```python
from build123d import *

# Parameters (mm, degrees)
F1_DEPTH = 22
F2_R     = 6
F3_W     = 66
F3_H     = 4
F4_DEPTH = 96
F5_R     = 4.6734146419
F5_R_2   = 4.6518685429
F5_R_3   = 4.696387476
F5_R_4   = 4.5347148874
F5_R_5   = 2.5803932982
F5_R_6   = 2.1193315606
F5_R_7   = 2.8799856964
F5_R_8   = 3.6433218135
F5_R_9   = 1.5618927534
F5_R_10  = 1.780828752
F5_R_11  = 1.3177092187
F5_R_12  = 1.8635222484
F5_R_13  = 1.68135752
F5_R_14  = 2.1595766427
F5_R_15  = 1.0781288147
F5_R_16  = 1.4474492092
F5_R_17  = 2.7862850737
F5_R_18  = 3.4582862602
F5_R_19  = 1.9500679084
F5_R_20  = 1.1979173869
F5_R_21  = 1.4573267426
F5_R_22  = 1.0781294395
F5_R_23  = 0.5989588797
F5_R_24  = 3.4929735647
F5_R_25  = 4.0355453194
F5_R_26  = 5.1927529479
F5_R_27  = 2.3790588204
F5_R_28  = 2.1982450571
F5_R_29  = 3.4468016913
F5_R_30  = 2.7968598425
F5_R_31  = 1.4614439331
F5_R_32  = 1.3473825629
F5_R_33  = 1.6339413822
F5_R_34  = 1.9124784447
F5_R_35  = 1.6663004851
F5_R_36  = 1.3473821111
F5_R_37  = 1.521199858
F5_R_38  = 1.189529666
F5_R_39  = 0.9803697467
F5_R_40  = 0.8958556794
F5_R_41  = 0.9362344169
F5_R_42  = 0.9000294175
F5_R_43  = 1.5546857265
F5_R_44  = 1.0528691723
F5_R_45  = 0.9573948707
F5_R_46  = 1.0252641854
F5_R_47  = 0.8253231645
F5_R_48  = 0.6675992995
F5_R_49  = 0.9215911414
F6_DEPTH = 19.0993858407


# Not quite as in the source:
# - a feature names something its author has since deleted; it is built from what else it names


with BuildPart() as f1:
    # F0 (on Top) → F1 (new body)
    with BuildSketch(Plane.XY):
        Polygon((9.8717576678, 17.0983858407), (-9.8717576678, 17.0983858407), (-19.7435153356, 0), (-9.8717576678, -17.0983858407), (9.8717576678, -17.0983858407), (19.7435153356, 0), align=None)
    extrude(amount=F1_DEPTH)

    # F2
    f2_edges = [f1.edges().sort_by_distance(p)[0] for p in [
        (14.807637, 8.549193, 22),
        (0, 17.098386, 22),
        (-14.807637, 8.549193, 22),
        (-14.807637, -8.549193, 22),
        (0, -17.098386, 22),
        (14.807637, -8.549193, 22),
    ]]
    fillet(f2_edges, radius=F2_R)

    # F3 (on face) → F4 (join)
    with BuildSketch(Plane.XY.offset(22)):
        Rectangle(F3_W, F3_H)
    extrude(amount=F4_DEPTH)

    # F5 (on face) → F6 (cut, through all)
    with BuildSketch(Plane.XZ.offset(2)):
        with Locations((-15.4567928985, 62.7651289105)):
            Circle(F5_R)
        with Locations((-8.0297058448, 52.103664726)):
            Circle(F5_R_2)
        with Locations((-5.9932461008, 39.0463657677)):
            Circle(F5_R_3)
        with Locations((5.7463436387, 37.3692810535)):
            Circle(F5_R_4)
        with Locations((4.9078003503, 45.8744950593)):
            Circle(F5_R_5)
        with Locations((9.4598866999, 49.7078299522)):
            Circle(F5_R_6)
        with Locations((9.6994703636, 55.8172091842)):
            Circle(F5_R_7)
        with Locations((18.3244738728, 58.6922094226)):
            Circle(F5_R_8)
        with Locations((18.3244738728, 64.6817982197)):
            Circle(F5_R_9)
        with Locations((14.2515562475, 53.4213744104)):
            Circle(F5_R_10)
        with Locations((-3.7172031589, 46.8328297138)):
            Circle(F5_R_11)
        with Locations((-10.185956955, 45.5151200294)):
            Circle(F5_R_12)
        with Locations((-9.467205964, 59.0515844524)):
            Circle(F5_R_13)
        with Locations((-15.0974178687, 55.3380399942)):
            Circle(F5_R_14)
        with Locations((-22.2849212587, 66.4786696434)):
            Circle(F5_R_15)
        with Locations((-17.0140843838, 69.9526295066)):
            Circle(F5_R_16)
        with Locations((-6.9515802898, 30.6609440595)):
            Circle(F5_R_17)
        with Locations((0, 30.3015690297)):
            Circle(F5_R_18)
        with Locations((5.5067595094, 24.0724012256)):
            Circle(F5_R_19)
        with Locations((5.3869681433, 29.5828189701)):
            Circle(F5_R_20)
        with Locations((-4.0765781887, 24.0724012256)):
            Circle(F5_R_21)
        with Locations((0, 24.0724012256)):
            Circle(F5_R_22)
        with Locations((-6.9515802898, 26.2286514044)):
            Circle(F5_R_23)
        with Locations((-20.7141488791, 110.4762628675)):
            Circle(F5_R_24)
        with Locations((-24.7990079224, 100.1824140549)):
            Circle(F5_R_25)
        with Locations((-23.4918538481, 77.6339918375)):
            Circle(F5_R_26)
        with Locations((-27.0865298808, 86.6206809878)):
            Circle(F5_R_27)
        with Locations((21.1148075759, 69.3008825183)):
            Circle(F5_R_28)
        with Locations((23.5657226294, 76.980419457)):
            Circle(F5_R_29)
        with Locations((22.2585685551, 90.3787538409)):
            Circle(F5_R_30)
        with Locations((22.585356608, 100.3458127379)):
            Circle(F5_R_31)
        with Locations((26.3434294611, 97.8948995471)):
            Circle(F5_R_32)
        with Locations((21.6049905866, 95.7707688212)):
            Circle(F5_R_33)
        with Locations((25.5264546722, 84.0063765645)):
            Circle(F5_R_34)
        with Locations((-24.9624028802, 93.1564569473)):
            Circle(F5_R_35)
        with Locations((-17.7730508149, 83.6795866489)):
            Circle(F5_R_36)
        with Locations((-21.2043337524, 70.2812448144)):
            Circle(F5_R_37)
        with Locations((-22.1846997738, 84.9867388606)):
            Circle(F5_R_38)
        with Locations((-18.916811794, 104.7574579716)):
            Circle(F5_R_39)
        with Locations((-30.0772096962, 116.170220077)):
            Circle(F5_R_40)
        with Locations((-26.9252173603, 113.7220710516)):
            Circle(F5_R_41)
        with Locations((-24.3240576237, 114.1811013222)):
            Circle(F5_R_42)
        with Locations((-25.8235502988, 106.8672537804)):
            Circle(F5_R_43)
        with Locations((22.332961016, 65.5509606004)):
            Circle(F5_R_44)
        with Locations((17.0422960073, 67.5684064627)):
            Circle(F5_R_45)
        with Locations((25.0203702599, 71.9701051712)):
            Circle(F5_R_46)
        with Locations((22.0859050751, 62.7999007702)):
            Circle(F5_R_47)
        with Locations((12.6406000927, 59.7737394273)):
            Circle(F5_R_48)
        with Locations((29.8805739731, 98.1968715787)):
            Circle(F5_R_49)
        Polygon((-11.660611567, 22), (-6.8317884579, 22), (-11.660611567, 31.6260260755), (-12.9401380399, 41.5687402004), (-14.4974304566, 48.5166599268), (-21.445350183, 62.1729185099), (-31.6276470402, 75.8291770929), (-30.214605853, 81.9581896067), (-31.6276470402, 88.4158834815), (-30.3520038724, 95.8353579044), (-30.3520038724, 101.1938676238), (-28.0701080944, 105.5646776068), (-27.4666510522, 109.5751300454), (-33, 118), (-33, 22), align=None)
        Polygon((33, 118), (-33, 118), (-15.0963891501, 114.3840551376), (-18.3763280511, 101.0725870728), (-22.5977953523, 90.0094285607), (-13.8637246564, 84.4778493047), (-13.8637246564, 72.1045807004), (-2.3638659623, 56.0921244323), (0, 40.8702604473), (1.6708788462, 50.837315619), (7.8798653558, 61.1311607063), (11.4745413885, 61.1311607063), (18.1737095118, 73.875926435), (20.6246245652, 83.6795866489), (16.0495843738, 94.7903990746), (22.2585685551, 105.0842478871), (33, 98.6052934028), align=None)
        Polygon((8.980720304, 30.9005267918), (8.980720304, 22), (11.660611567, 22), (33, 22), (33, 98.6052934028), (28.467554599, 94.9537977576), (26.3434294611, 91.9126495719), (30.7337772995, 82.5414285064), (27.1243248135, 70.3275278211), (22.332961016, 56.0962293618), (10.1786367595, 43.5984507203), (13.2932206616, 36.6505309939), align=None)
    extrude(amount=-F6_DEPTH, mode=Mode.SUBTRACT)


solid = f1.part
```
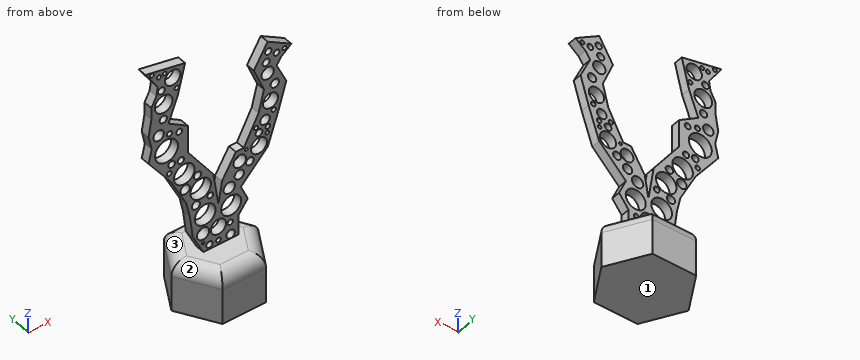
The model under review builds one solid part; all positions refer to its coordinate system, in mm. Face numbers are marked on the shaded views. A direction names the side the tool comes from. Round coordinates to 2 decimals unless told otherwise and drop trailing zeros. Answer in a Markdown table with one row per item.
(1) Clearance check with flat-ended pins moving along their axes: P1, Ø6.5, axis at x = 4.91, z = 45.87, coming from the -Y side; P2, Ø10, axis at x = 8, y = 0.5, coming from the +Z side; P3, Ø6, axis at y = -1, z = 65.5, coming from the +X side. State where each tip first meets the part, or that it passes through.
Result set:
| item | result |
|---|---|
| P1 | stops at y = -2 |
| P2 | stops at z = 64.03 |
| P3 | stops at x = 26.51 |
(2) Machinability: for the marked faces 1, 2 and 3, which of the approach directions +Z, -Z, +X, -X, +Y, -Y give a long, thin tool a straight path to every point of the face, cutting with its end or side? Answer none if there is none.
Result set:
| item | result |
|---|---|
| face 1 | -Z, +X, -X, +Y, -Y |
| face 2 | -X, -Y |
| face 3 | -X, +Y |
(3) For line 1 (X direction, y = 0, z = 76.5); line 2 (Y direction, x = 15, z = 55.5); line 3 (Z direction, x = -7, y = 8.5), list the stretches that pass through material, from the lowest coordinate up. Write a range as from..to.
Result set:
| item | result |
|---|---|
| line 1 | x = -31.47..-28.56, -18.42..-13.86, 18.83..20.15, 26.98..28.95 |
| line 2 | y = -2..2 |
| line 3 | z = 0..22 |
